Study the drawing (mm; zero at the part's minimum x, y, z) and answer. A direction names the side the tool comes from. Give positions to 0.01 mm unless a question says otherwise; leave off trailing zeros. Order: outer loops, then holes, each group sorted by start corner. A loop starts at its lowest first (then second) coordinate and runs counter-clockwise, first axis right, second up. Notation, with made-up numbers: (24.25, 56) - (29.25, 56) arc R34 cw to (29.25, 93) - close; hole circle Ø4 at (-34, -18). An arc over 180 degrees is marked (long way). Return JSON: item names as keys, results as strings.
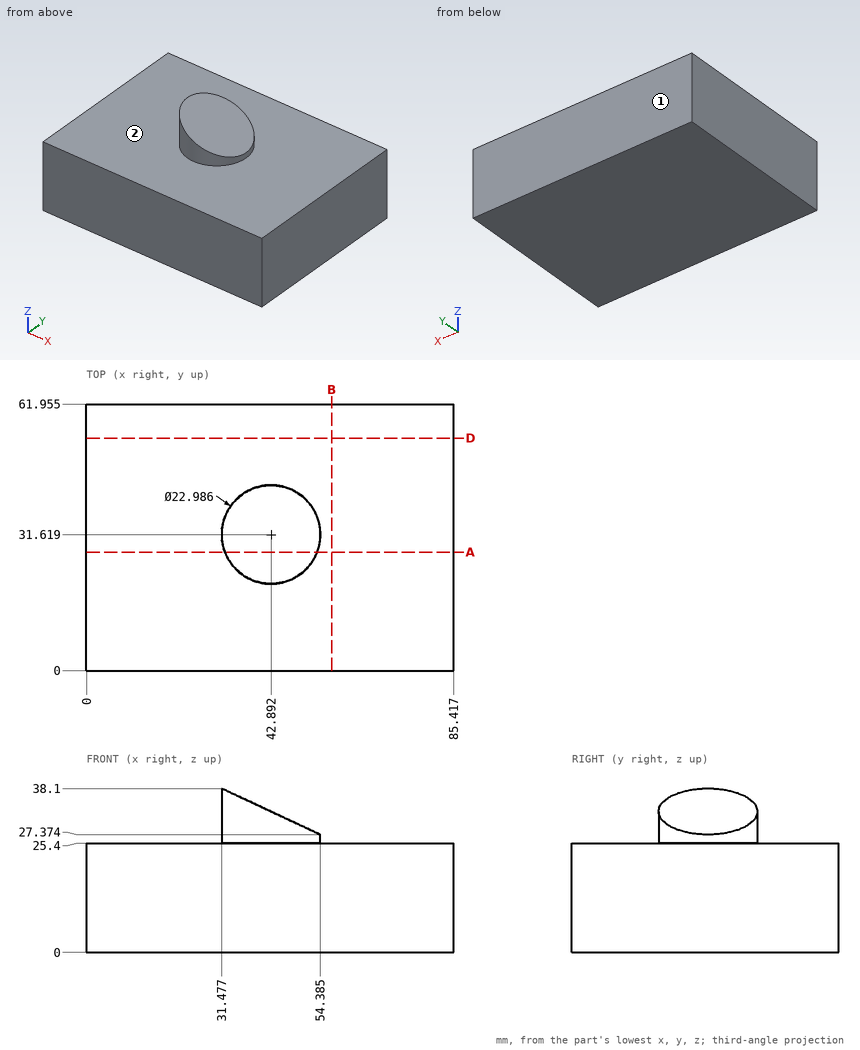
Q1. Consider L1, parallel to Z at x = 69.5, y = 39; L2, parallel to Z at x = 42, y = 42.5; L3, parallel to X at y = 25, z = 26 (1 decimal). Determine where each line is inside the solid, lowest interval first.
Values:
{"L1": "z = 0 to 25.4", "L2": "z = 0 to 33.17", "L3": "x = 33.5 to 52.3"}
Q2. A cutting plane is placed at D-D (y = 54). Write down the section's boundary in (x, z), and give its area (3 significant figures).
Values:
{"outline": "(0, 0) - (85.42, 0) - (85.42, 25.4) - (0, 25.4) - close", "area": "2,170 mm²"}
Q3. Given pin 1 (4 mm diameter, centred on y = 43.5, z = 24.5, fed in from -X); pin 2 (18.5 mm diameter, centred on x = 61.5, y = 36.5, fed in from +Z); pin 3 (12 mm diameter, centred on x = 47, y = 42, fed in from +Z), each flat-ended and moving along its own axis, determine where each tip first touches the part or whether it passes through.
Values:
{"pin 1": "stops at x = 0", "pin 2": "stops at z = 28.37", "pin 3": "stops at z = 33.64"}
Q4. For the marked faces 1 and 2, determine the directions among +Z, -Z, +X, -X, +Y, -Y from which every point of the face is accessible in a straight line to the end or side of a thin tool.
Values:
{"face 1": "+Z, -Z, +X, -X, +Y", "face 2": "+Z"}
Q5. A cutting plane is placed at A-A (y = 27.5). Write down the section's boundary in (x, z).
Values:
{"outline": "(0, 0) - (85.42, 0) - (85.42, 25.4) - (53.62, 25.4) - (53.62, 27.73) - (32.16, 37.78) - (32.16, 25.4) - (0, 25.4) - close"}
Q6. A cutting plane is placed at B-B (x = 57). Write down the section's boundary in (y, z) (1 decimal).
Values:
{"outline": "(0, 0) - (62, 0) - (62, 25.4) - (0, 25.4) - close"}
